from build123d import *

# Parameters (mm, degrees)
SZKIC1_R                    = 2.5
SZKIC1_R_2                  = 0.75
DODANIE_WYCI_GNI_CIE1_DEPTH = 2.5


with BuildPart() as part:
    # Szkic1 → Dodanie-wyciągnięcie1 (new body)
    with BuildSketch(Plane.XY):
        with BuildLine():
            Line((-12.5, 34), (-12.5, 0))
            Line((-12.5, 0), (12.5, 0))
            Line((12.5, 0), (12.5, 34))
            ThreePointArc((12.5, 34), (0, 46.5), (-12.5, 34))
        make_face()
        with Locations((0, 34)):
            Circle(SZKIC1_R, mode=Mode.SUBTRACT)
        with Locations((0, 39.656854249)):
            Circle(SZKIC1_R_2, mode=Mode.SUBTRACT)
        with Locations((5.656854249, 34)):
            Circle(SZKIC1_R_2, mode=Mode.SUBTRACT)
        with Locations((0, 28.343145751)):
            Circle(SZKIC1_R_2, mode=Mode.SUBTRACT)
        with Locations((-5.656854249, 34)):
            Circle(SZKIC1_R_2, mode=Mode.SUBTRACT)
        with BuildLine():
            Line((-3, 23), (-3, 8))
            ThreePointArc((-3, 8), (-6.5, 4.5), (-10, 8))
            Line((-10, 8), (-10, 23))
            ThreePointArc((-10, 23), (-6.5, 26.5), (-3, 23))
        make_face(mode=Mode.SUBTRACT)
        with BuildLine():
            Line((3, 23), (3, 8))
            ThreePointArc((3, 8), (6.5, 4.5), (10, 8))
            Line((10, 8), (10, 23))
            ThreePointArc((10, 23), (6.5, 26.5), (3, 23))
        make_face(mode=Mode.SUBTRACT)
    extrude(amount=DODANIE_WYCI_GNI_CIE1_DEPTH)


solid = part.part
The listing builds one solid part. Answer for the finished solid, in the listing's coordinates (mm). A direction names the side the tool comes from. Round coordinates to 2 decimals unless told otherwise and drop trailing zeros. Loops run counter-clockwise (first coordinate to the right, second up) from the corner with the lowest first, then second, coordinate; pieces in that order, holes last. Notation, with made-up numbers: M 14.25,-18.75 L 69.25,-18.75 A17 cw 69.25,-14.75 Z; hole C 38,-29.5 d4. An arc over 180 degrees is marked long. Write each question's results on one line, items separated by ' | '. Start each with the question number.
1) Which of the six approach directions +Z, -Z, +X, -X, +Y, -Y give full straight-line access (tool end or side, diameter ignored) to faces 5 (the cylindrical face through (0.275, 46.497, 1.232)), 6 (the cylindrical face through (6.4, 4.5, 1.2))?
2) Find section B-B on x = 0. Write down the section's boundary in (y, z).
3) Determine the mould class of faces 1 (the flat face through (12.5, 17, 1)), 2 (the cylindrical face through (1.34, 36.11, 1.23)), 3 (the flat face through (0, 0, 1)), 4 (the cylindrical face through (6.6, 26.5, 1.2)) for opening direction X: pulls with the +X half, pulls with the -X half, needs draft (parallel to the pull), parting line crosses it, or undercut.
4) Straight lines are drawn through the part: probe 1 along X at (y, z) = (15, 2); probe 2 along Y at (x, z) = (0, 0.75); probe 3 along X at (y, z) = (7, 1.5). For each, find the intervals that lie inside material, in ascending order.
5) Find section A-A on y = 13. Write down the section's boundary in (x, z).
6) Find section D-D on z = 1.65. Write down the section's boundary in (x, y), plus the area to 3 significant figures.
7) Find section C-C on x = 4. Write down the section's boundary in (y, z).
Final values:
1) face 5: +Z, -Z, +Y | face 6: +Z, -Z
2) outline: M 0,0 L 27.59,0 L 27.59,2.5 L 0,2.5 Z; M 29.09,0 L 31.5,0 L 31.5,2.5 L 29.09,2.5 Z; M 36.5,0 L 38.91,0 L 38.91,2.5 L 36.5,2.5 Z; M 40.41,0 L 46.5,0 L 46.5,2.5 L 40.41,2.5 Z
3) face 1: pulls with the +X half | face 2: undercut | face 3: needs draft | face 4: undercut
4) probe 1: -12.5 to -10, -3 to 3, 10 to 12.5 | probe 2: 0 to 27.59, 29.09 to 31.5, 36.5 to 38.91, 40.41 to 46.5 | probe 3: -12.5 to -9.85, -3.15 to 3.15, 9.85 to 12.5
5) outline: M -12.5,0 L -10,0 L -10,2.5 L -12.5,2.5 Z; M -3,0 L 3,0 L 3,2.5 L -3,2.5 Z; M 10,0 L 12.5,0 L 12.5,2.5 L 10,2.5 Z
6) outline: M -12.5,0 L 12.5,0 L 12.5,34 A12.5 ccw -12.5,34 Z; hole M -10,8 A3.5 ccw -3,8 L -3,23 A3.5 ccw -10,23 Z; hole C -5.66,34 d1.5; hole C 0,34 d5; hole C 0,28.34 d1.5; hole C 0,39.66 d1.5; hole M 3,8 A3.5 ccw 10,8 L 10,23 A3.5 ccw 3,23 Z; hole C 5.66,34 d1.5 | area: 782 mm²
7) outline: M 0,0 L 5.55,0 L 5.55,2.5 L 0,2.5 Z; M 25.45,0 L 45.84,0 L 45.84,2.5 L 25.45,2.5 Z
